from build123d import *

# Parameters (mm, degrees)
EXTRUDE_1_DEPTH     = 10
SKETCH_2_R          = 2.55
CUT_EXTRUDE_1_DEPTH = 19
CUT_EXTRUDE_2_DEPTH = 19
SKETCH_5_W          = 10
SKETCH_5_H          = 2
CUT_EXTRUDE_4_DEPTH = 19
SKETCH_6_R          = 6.3
CUT_EXTRUDE_5_DEPTH = 19
CUT_EXTRUDE_6_DEPTH = 19
SKETCH_8_R          = 1
CUT_EXTRUDE_7_DEPTH = 18


with BuildPart() as part:
    # 草图1 → 凸台-拉伸1 (new body)
    with BuildSketch(Plane.XY):
        Polygon((0, 0), (35, 0), (35, -3.5), (47, -3.5), (47, -6.5), (35, -6.5), (35, -9.5), (47, -9.5), (47, -12.5), (35, -12.5), (35, -15.5), (47, -15.5), (47, -18.5), (35, -18.5), (35, -22), (0, -22), (0, -17), (-10, -17), (-10, -12), (0, -12), (0, -10), (-10, -10), (-10, -5), (0, -5), align=None)
    extrude(amount=EXTRUDE_1_DEPTH)

    # 草图2 → 切除-拉伸1 (cut)
    with BuildSketch(Plane(origin=(0, -3.5, 0), x_dir=(1, 0, 0), z_dir=(0, 1, 0))):
        with Locations((42, -5)):
            Circle(SKETCH_2_R)
    extrude(amount=-CUT_EXTRUDE_1_DEPTH, mode=Mode.SUBTRACT)

    # 草图3 → 切除-拉伸2 (cut)
    with BuildSketch(Plane(origin=(0, -3.5, 0), x_dir=(1, 0, 0), z_dir=(0, 1, 0))):
        with BuildLine():
            Line((42, 0), (35, 0))
            Line((35, 0), (35, 1.362905895))
            Line((35, 1.362905895), (53.328864927, 1.362905895))
            Line((53.328864927, 1.362905895), (53.328864927, -13.813237877))
            Line((53.328864927, -13.813237877), (35, -13.813237877))
            Line((35, -13.813237877), (35, -10))
            Line((35, -10), (42, -10))
            ThreePointArc((42, -10), (47, -5), (42, 0))
        make_face()
    extrude(amount=-CUT_EXTRUDE_2_DEPTH, mode=Mode.SUBTRACT)

    # 草图5 → 切除-拉伸4 (cut)
    with BuildSketch(Plane.XY.offset(10)):
        with Locations((5, -11)):
            Rectangle(SKETCH_5_W, SKETCH_5_H)
    extrude(amount=-CUT_EXTRUDE_4_DEPTH, mode=Mode.SUBTRACT)

    # 草图6 → 切除-拉伸5 (cut)
    with BuildSketch(Plane.XY.offset(10)):
        with Locations((10, -11)):
            Circle(SKETCH_6_R)
    extrude(amount=-CUT_EXTRUDE_5_DEPTH, mode=Mode.SUBTRACT)

    # 草图7 → 切除-拉伸6 (cut)
    with BuildSketch(Plane(origin=(0, -5, 0), x_dir=(1, 0, 0), z_dir=(0, 1, 0))):
        with BuildLine():
            Line((-4.422847497, -10), (-4.422847497, -16.245470045))
            Line((-4.422847497, -16.245470045), (-15.241663488, -16.245470045))
            Line((-15.241663488, -16.245470045), (-15.241663488, 3.326156632))
            Line((-15.241663488, 3.326156632), (-3, 3.326156632))
            Line((-3, 3.326156632), (-3, 0))
            ThreePointArc((-3, 0), (-5.308519262, -4.772757665), (-4.422847497, -10))
        make_face()
    extrude(amount=-CUT_EXTRUDE_6_DEPTH, mode=Mode.SUBTRACT)

    # 草图8 → 切除-拉伸7 (cut)
    with BuildSketch(Plane(origin=(0, -5, 0), x_dir=(1, 0, 0), z_dir=(0, 1, 0))):
        with Locations((-2.5, -6)):
            Circle(SKETCH_8_R)
    extrude(amount=-CUT_EXTRUDE_7_DEPTH, mode=Mode.SUBTRACT)


solid = part.part
Verification items for the finished model (mm, model axes). A direction names the side the tool comes from. Round coordinates to 2 decimals unless told otherwise and drop trailing zeros. Loops run counter-clockwise (first coordinate to the right, second up) from the corner with the lowest first, then second, coordinate; pieces in that order, holes last. Notation, with made-up numbers: (89, 25.25) - (106, 25.25) arc R14 ccw to (106, 38.25) - close; hole circle Ø4 at (-14.5, -26.5). An arc over 180 degrees is marked (long way). Use a Markdown table: item, result. Add a question column.
1. Gauge pin test, flat ends, axial feed: pin 1 (6 mm diameter, centred on y = -5.5, z = 3.5, fed in from +X); pin 2 (0.9 mm diameter, centred on y = -8, z = 6.5, fed in from +X); pin 3 (1.6 mm diameter, centred on x = -3.5, z = 4.5, fed in from +Y); pin 4 (3 mm diameter, centred on x = 38, z = 4.5, fed in from -Y). Record the tip position at first contact, or that the pin passes through.
2. Section check C-C, the plane x = 10. Record the boundary of the cut face in (y, z).
3. Access from +Z, -Z, +X, -X, +Y, -Y to the whole of each face (thin tool, end or side, straight path). Record for faces 4 (the face through (38, -3.5, 5)), 5 (the face through (35, -20, 5)), 6 (the face through (-2.1, -5, 4.9)).
4. Section check B-B, the plane y = -13.75. Record the boundary of the cut face in (x, z).
5. Section check D-D, the plane y = -11. Record the boundary of the cut face in (x, z).
6. Thickness scan on probe 1 along Y at (x, z) = (39.5, 7.25); probe 2 along Z at (x, y) = (42, -5.55); probe 3 along Z at (x, y) = (-2.5, -7.5). Record the ranges inside material, lowest first. Write a range as [from, to].
7. Release check for a two-part mould opening along Y. For faces 1 (the face through (38, -9.5, 5)), 2 (the face through (17, 0, 5)), 3 (the face through (47, -17, 5)) record: released by +Y, released by -Y, zero draft, split by the parting line, or undercut.
8. Section check A-A, the plane x = 36. Record the boundary of the cut face in (y, z).
Checks:
| question | item | result |
|---|---|---|
| 1 | pin 1 | stops at x = 47 |
| 1 | pin 2 | stops at x = 35 |
| 1 | pin 3 | stops at y = -5 |
| 1 | pin 4 | stops at y = -18.5 |
| 2 | outline | (-22, 0) - (-17.3, 0) - (-17.3, 10) - (-22, 10) - close; (-4.7, 0) - (0, 0) - (0, 10) - (-4.7, 10) - close |
| 3 | face 4 | +Z, -Z, +X, +Y |
| 3 | face 5 | +Z, -Z, +X, -Y |
| 3 | face 6 | +Z, -Z, -X, +Y |
| 4 | outline | (-4.42, 10) arc R8.71 ccw to (-3, 0) - (4.33, 0) - (4.33, 10) - close; (15.67, 0) - (35, 0) - (35, 10) - (15.67, 10) - close; hole circle Ø2 at (-2.5, 6) |
| 5 | outline | (16.3, 0) - (42, 0) arc R5 ccw to (42, 10) - (16.3, 10) - close; hole circle Ø5.1 at (42, 5) |
| 6 | probe 1 | y = [-18.5, -15.5], [-12.5, -9.5], [-6.5, -3.5] |
| 6 | probe 2 | z = [0, 2.45], [7.55, 10] |
| 6 | probe 3 | z = [0, 5], [7, 10] |
| 7 | face 1 | undercut |
| 7 | face 2 | released by +Y |
| 7 | face 3 | zero draft |
| 8 | outline | (-18.5, 0) - (-15.5, 0) - (-15.5, 10) - (-18.5, 10) - close; (-12.5, 0) - (-9.5, 0) - (-9.5, 10) - (-12.5, 10) - close; (-6.5, 0) - (-3.5, 0) - (-3.5, 10) - (-6.5, 10) - close |
